from build123d import *

# Parameters (mm, degrees)
BOSS_EXTRUDE1_DEPTH = 61.5
SKETCH3_R           = 17.5
BOSS_EXTRUDE2_DEPTH = 4.7
SKETCH4_W           = 14.228114438
SKETCH4_H           = 15.553065114
BOSS_EXTRUDE3_DEPTH = 6.3


with BuildPart() as part:
    # Sketch1 → Boss-Extrude1 (new body)
    with BuildSketch(Plane.XY):
        with BuildLine():
            Line((2.7, 0), (34.3, 0))
            ThreePointArc((34.3, 0), (36.209188309, 0.790811691), (37, 2.7))
            Line((37, 2.7), (37, 34.3))
            ThreePointArc((37, 34.3), (36.209188309, 36.209188309), (34.3, 37))
            Line((34.3, 37), (2.7, 37))
            ThreePointArc((2.7, 37), (0.790811691, 36.209188309), (0, 34.3))
            Line((0, 34.3), (0, 2.7))
            ThreePointArc((0, 2.7), (0.790811691, 0.790811691), (2.7, 0))
        make_face()
    extrude(amount=BOSS_EXTRUDE1_DEPTH)

    # Sketch3 → Boss-Extrude2 (add)
    with BuildSketch(Plane.XY.offset(61.5)):
        with Locations((18.5, 18.5)):
            Circle(SKETCH3_R)
    extrude(amount=BOSS_EXTRUDE2_DEPTH)

    # Sketch4 → Boss-Extrude3 (add)
    with BuildSketch(Plane(origin=(0, 0, 0), x_dir=(-1, 0, 0), z_dir=(0, 0, -1))):
        with Locations((-12.194929465, 22.979733571)):
            Rectangle(SKETCH4_W, SKETCH4_H)
    extrude(amount=BOSS_EXTRUDE3_DEPTH)


solid = part.part
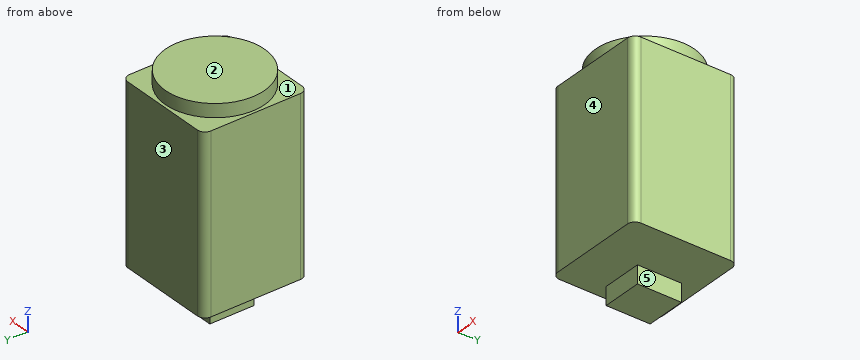
Here's how the part is built. I have some questions about the finished solid (model axes, mm). Face numbers are marked on the shaded views. A direction names the side the tool comes from. Coordinates: 2 decimals unless noted, no trailing zeros. Order: outer loops, then holes, each group sorted by start corner. A loop starts at its lowest first (then second) coordinate and runs counter-clockwise, first axis right, second up. Notation, with made-up numbers: M -21,-11 L 37,-11 A18 ccw 37,18 Z; hole C -17.75,50 d11. An arc over 180 degrees is marked long. Answer as CSV lines item,"result".
Item 1: Imagine slicing it at D-D on x = 33.5. Write out the boundary of the cut face in (y, z).
Results found:
outline,"M 0,0 L 37,0 L 37,61.5 L 27.51,61.5 L 27.51,66.2 L 9.49,66.2 L 9.49,61.5 L 0,61.5 Z"
Item 2: We'd pull the mould along Y, two halves only. Please class the marked faces 3, 4 and 5: +Y half, -Y half, draft (parallel to the pull), parting line (faces both ways), or undercut.
Results found:
face 3,"+Y half"
face 4,"-Y half"
face 5,"draft"
Item 3: For pin 1 (7 mm diameter, centred on x = 11.5, z = -4.5, fed in from +Y); pin 2 (3 mm diameter, centred on y = 20.5, z = -3.5, fed in from -X); pin 3 (3 mm diameter, centred on y = 21.5, z = -3, fed in from +X); pin 4 (11 mm diameter, centred on x = 23, y = 27, fed in from -Z), each with a flat end and sliding along its axis, tell me the tip position at first contact or that it passes through.
Results found:
pin 1,"y = 30.76"
pin 2,"x = 5.08"
pin 3,"x = 19.31"
pin 4,"z = -6.3"
Item 4: If I drill on line 1 (Z direction, x = 15.5, y = 6.5); line 2 (Y direction, x = 2.5, z = 37); line 3 (Z direction, x = 29.5, y = 2), over which ranges is the centre line in solid material (lowest first)?
Results found:
line 1,"0 to 66.2"
line 2,"0.01 to 36.99"
line 3,"0 to 61.5"
Item 5: Imagine slicing it at A-A on x = 18.5. Write out the boundary of the cut face in (y, z), plus the area to 3 significant figures.
Results found:
outline,"M 0,0 L 15.2,0 L 15.2,-6.3 L 30.76,-6.3 L 30.76,0 L 37,0 L 37,61.5 L 36,61.5 L 36,66.2 L 1,66.2 L 1,61.5 L 0,61.5 Z"
area,"2,540 mm2"
Item 6: Imagine slicing it at B-B on y = 18.5. Write out the boundary of the cut face in (x, z).
Results found:
outline,"M 0,0 L 5.08,0 L 5.08,-6.3 L 19.31,-6.3 L 19.31,0 L 37,0 L 37,61.5 L 36,61.5 L 36,66.2 L 1,66.2 L 1,61.5 L 0,61.5 Z"
Item 7: On a 3-axis mill with a long thin cutter (end or side, diameter ignored), from which of +Z, -Z, +X, -X, +Y, -Y can I reach the whole of each face in a straight line? I mean the marked faces 1 and 2. Say none if no direction works.
Results found:
face 1,"+Z"
face 2,"+Z, +X, -X, +Y, -Y"
Item 8: Imagine slicing it at C-C on y = 32. Write out the boundary of the cut face in (x, z).
Results found:
outline,"M 0,0 L 37,0 L 37,61.5 L 29.64,61.5 L 29.64,66.2 L 7.36,66.2 L 7.36,61.5 L 0,61.5 Z"
